from build123d import *

# Parameters (mm, degrees)
SKETCH1_W                = 135
SKETCH1_H                = 20
BOSS_EXTRUDE1_DEPTH      = 3
BOSS_EXTRUDE2_START      = -20
BOSS_EXTRUDE2_DEPTH      = 20
SKETCH5_R                = 1.6
CUT_EXTRUDE1_DEPTH       = 5
BOSS_EXTRUDE3_DEPTH      = 2.7
SKETCH7_W                = 5
SKETCH7_H                = 2.576431393
BOSS_EXTRUDE4_DEPTH      = 20
SKETCH9_W                = 5
SKETCH9_H                = 2.400677448
SKETCH9_H_2              = 2.137863312
BOSS_EXTRUDE5_DEPTH      = 18
SKETCH10_R               = 1.51
CUT_EXTRUDE2_DEPTH       = 46
SKETCH11_W               = 87
SKETCH11_H               = 20
CUT_EXTRUDE3_DEPTH       = 7
BOSS_EXTRUDE7_DEPTH      = 26.162
BOSS_EXTRUDE7_DEPTH_BACK = 3
SKETCH12_W               = 9.518804698
SKETCH12_H               = 20
SKETCH13_R               = 1.6
CUT_EXTRUDE4_DEPTH       = 36.162
BOSS_EXTRUDE8_DEPTH      = 4
FILLET1_R                = 10
SKETCH18_R               = 1.6
CUT_EXTRUDE6_DEPTH       = 4


# Read off the part's stored shape, not the designer's step: Boss-Extrude2
with BuildPart() as part:
    # Sketch1 → Boss-Extrude1 (new body)
    with BuildSketch(Plane(origin=(0, 0, 0), x_dir=(1, 0, 0), z_dir=(0, 1, 0))):
        with Locations((67.5, 10)):
            Rectangle(SKETCH1_W, SKETCH1_H)
    extrude(amount=BOSS_EXTRUDE1_DEPTH)


with BuildPart() as body_2:
    # Boss-Extrude2 outline → Boss-Extrude2 (new body)
    with BuildSketch(Plane(origin=(0, 0, -20), x_dir=(-1, 0, 0), z_dir=(0, 0, -1)).offset(BOSS_EXTRUDE2_START)):
        Polygon((-135, 0), (0, 0), (0, -26.161397266), (8, -26.161397266), (8, -23.458863774), (2.440744198, -23.458863774), (2.440744198, 3), (-135, 3), align=None)
    extrude(amount=BOSS_EXTRUDE2_DEPTH)

    # Sketch5 → Cut-Extrude1 (cut)
    with BuildSketch(Plane(origin=(0, -26.161397266, 0), x_dir=(-1, 0, 0), z_dir=(0, -1, 0))):
        with Locations(Location((4.475005096, 14.904630263, 0), (0, 0, 90))):
            Circle(SKETCH5_R)
        with Locations(Location((4.475005096, 4.904630263, 0), (0, 0, 90))):
            Circle(SKETCH5_R)
    extrude(amount=-CUT_EXTRUDE1_DEPTH, mode=Mode.SUBTRACT)

    # Sketch6 → Boss-Extrude3 (add)
    with BuildSketch(Plane(origin=(0, -26.161397266, 0), x_dir=(-1, 0, 0), z_dir=(0, -1, 0))):
        Polygon((0, 26.189005721), (0, 20), (8, 20), (8, 23.612574328), (17, 23.612574328), (17, 26.189005721), align=None)
    extrude(amount=-BOSS_EXTRUDE3_DEPTH)

    # Sketch7 → Boss-Extrude4 (add)
    with BuildSketch(Plane.XZ.offset(26.161397266)):
        with Locations((-14.5, -24.900790025)):
            Rectangle(SKETCH7_W, SKETCH7_H)
    extrude(amount=BOSS_EXTRUDE4_DEPTH)

    # Sketch9 → Boss-Extrude5 (add)
    with BuildSketch(Plane.XY.offset(-23.612574328)):
        with Locations((-14.5, -44.961058542)):
            Rectangle(SKETCH9_W, SKETCH9_H)
        with Locations((-14.5, -37.813107102)):
            Rectangle(SKETCH9_W, SKETCH9_H_2)
    extrude(amount=BOSS_EXTRUDE5_DEPTH)

    # Sketch10 → Cut-Extrude2 (cut)
    with BuildSketch(Plane(origin=(0, -46.161397266, 0), x_dir=(-1, 0, 0), z_dir=(0, -1, 0))):
        with Locations(Location((14.400768804, 9.736347936, 0), (0, 0, 90))):
            Circle(SKETCH10_R)
    extrude(amount=-CUT_EXTRUDE2_DEPTH, mode=Mode.SUBTRACT)


with BuildPart() as cut_extrude3_tool:
    # Sketch11 → Cut-Extrude3 (new body)
    with BuildSketch(Plane.XZ):
        with Locations((91.5, -10)):
            Rectangle(SKETCH11_W, SKETCH11_H)
    extrude(amount=-CUT_EXTRUDE3_DEPTH)


with BuildPart() as part_1:
    add(part.part)

    # Cut-Extrude3: cut by cut_extrude3_tool
    add(cut_extrude3_tool.part, mode=Mode.SUBTRACT)



with BuildPart() as body_2_1:
    add(body_2.part)

    # Cut-Extrude3: cut by cut_extrude3_tool
    add(cut_extrude3_tool.part, mode=Mode.SUBTRACT)


with BuildPart() as part_2:
    add(part_1.part)

    add(body_2_1.part)  # Boss-Extrude7 merges body 2
    # Sketch12 → Boss-Extrude7 (add, two sides: drawn at the far end of the back side and taken through both)
    with BuildSketch(Plane(origin=(0, 0, 0), x_dir=(-1, 0, 0), z_dir=(0, -1, 0)).offset(-BOSS_EXTRUDE7_DEPTH_BACK)):
        with Locations((-45.240597651, 10)):
            Rectangle(SKETCH12_W, SKETCH12_H)
    extrude(amount=BOSS_EXTRUDE7_DEPTH + BOSS_EXTRUDE7_DEPTH_BACK)

    # Sketch13 → Cut-Extrude4 (cut)
    with BuildSketch(Plane(origin=(0, -26.162, 0), x_dir=(-1, 0, 0), z_dir=(0, -1, 0))):
        with Locations(Location((-45.024994904, 4.904630263, 0), (0, 0, 90))):
            Circle(SKETCH13_R)
        with Locations(Location((-45.024994904, 14.904630263, 0), (0, 0, 90))):
            Circle(SKETCH13_R)
    extrude(amount=-CUT_EXTRUDE4_DEPTH, mode=Mode.SUBTRACT)

    # Sketch14 → Boss-Extrude8 (add)
    with BuildSketch(Plane(origin=(0, 3, 0), x_dir=(1, 0, 0), z_dir=(0, 1, 0))):
        Polygon((50, 20), (50, 0), (148.480775301, 17.298817767), (148.480775301, 37.364817767), align=None)
    extrude(amount=-BOSS_EXTRUDE8_DEPTH)

    # Fillet1
    # the kernel refuses this fillet: 10 mm, written as the material it takes off along each edge
    with BuildSketch(Plane(origin=(148.480775301, 23.991341286, -17.298817767), x_dir=(-0.9849204245014849, 0, 0.1730079691800782), z_dir=(0, -1, 0))) as fillet1_piece_1:
        with BuildLine():
            CenterArc((FILLET1_R * 0.83965365145, FILLET1_R), FILLET1_R, 189.96275502, 80.03724498)
            Line((-FILLET1_R * 0.145266773052, FILLET1_R * 0.82699203082), (0, 0))
            Line((0, 0), (FILLET1_R * 0.83965365145, 0))
        make_face()
    extrude(amount=45.982682572, mode=Mode.SUBTRACT)
    with BuildSketch(Plane(origin=(148.480775301, 32.793839815, -37.364817767), x_dir=(0, 0, 1), z_dir=(0, -1, 0))) as fillet1_piece_2:
        with BuildLine():
            CenterArc((FILLET1_R * 1.19175359259, FILLET1_R), FILLET1_R, 170, 100)
            Line((FILLET1_R * 0.206945839582, FILLET1_R * 1.17364817767), (0, 0))
            Line((0, 0), (FILLET1_R * 1.19175359259, 0))
        make_face()
    extrude(amount=63.58767963, mode=Mode.SUBTRACT)

    # Sketch18 → Cut-Extrude6 (cut)
    with BuildSketch(Plane(origin=(0, 3, 0), x_dir=(1, 0, 0), z_dir=(0, 1, 0))):
        with Locations(Location((138.480775301, 25.447281841, 0), (0, 0, 270))):
            Circle(SKETCH18_R)
        with Locations(Location((119.473985668, 22.095872012, 0), (0, 0, 270))):
            Circle(SKETCH18_R)
        with Locations(Location((110.610715891, 20.533038413, 0), (0, 0, 270))):
            Circle(SKETCH18_R)
        with Locations(Location((129.617505524, 23.884448242, 0), (0, 0, 270))):
            Circle(SKETCH18_R)
    extrude(amount=-CUT_EXTRUDE6_DEPTH, mode=Mode.SUBTRACT)


solid = part_2.part
Could you check a few things on this model? Use its own coordinates, in mm. A direction names the side the tool comes from. Give positions to 0.01 mm unless a question says otherwise; leave off trailing zeros. Write each loop counter-clockwise with the first axis right and the second up, starting at its lowest first coordinate (ties: lowest second). Pieces come first, ordered by that corner, then holes. Notation, with made-up numbers: (86, 64.5) -> (112, 64.5) arc R11 cw to (112, 78.5) -> close; hole circle Ø5 at (53, 5). An arc over 180 degrees is marked (long way). Answer as a JSON object with one key per item and string values.
Q1. We'd pull the mould along Z, two halves only. Please class faces 4 (the cylindrical face through (144.8, 1, -33.2)), 5 (the flat face through (-14, -29, -23.613)), 6 (the cylindrical face through (130.1, 1.03, -22.36)): released by +Z, released by -Z, zero draft, split by the parting line, or undercut.
Taken from the geometry:
{"face 4": "released by -Z", "face 5": "released by +Z", "face 6": "undercut"}
Q2. Which directions (+Z, -Z, +X, -X, +Y, -Y) give clear straight access to the entire face, cutting with the end or side of a thin tool? Please do faces 1 (the flat face through (-5, -23.459, -10)), 2 (the flat face through (-6, -23.461, -24)), 3 (the flat face through (-12, -38, -18)).
Taken from the geometry:
{"face 1": "+Z, -Z, -X, +Y", "face 2": "-Z, +X, -X, +Y", "face 3": "+Z, -Z, +X, -Y"}
Q3. Suppose I cut it at B-B on x = 11.5. Write out the boundary of the cut face in (y, z), then the cut area to 3 significant figures.
Taken from the geometry:
{"outline": "(0, -20) -> (3, -20) -> (3, 0) -> (0, 0) -> close", "area": "60.0 mm²"}
Q4. Suppose I cut it at A-A on y = -21. Write out the boundary of the cut face in (x, z) (3 decimals), then the cut area to 3 significant figures.
Taken from the geometry:
{"outline": "(-2.441, -20) -> (0, -20) -> (0, 0) -> (-2.441, 0) -> close; (40.481, -20) -> (50, -20) -> (50, 0) -> (40.481, 0) -> close; hole circle Ø3.2 at (45.025, -14.905); hole circle Ø3.2 at (45.025, -4.905)", "area": "223 mm²"}
Q5. Will these pins go through, and if not, where does the flat tip stop? pin 1 Ø2 at (y, z) = (-39.5, -18.5) entering from +X; pin 2 Ø1.9 at (x, z) = (119.47, -22.1) entering from +Y; pin 3 Ø21 at (y, z) = (-7.5, -13.5) entering from +X; pin 4 Ø4 at (x, z) = (-13.5, -11.5) entering from +Y.
Taken from the geometry:
{"pin 1": "stops at x = -12", "pin 2": "passes through", "pin 3": "stops at x = 147.67", "pin 4": "stops at y = -36.74"}
Q6. Please list where these lines run through material, in increasing order: L1, parallel to X at y = -18, z = -1.5; L2, parallel to Y at x = -5.5, z = -10; L3, parallel to Y at x = 14.5, z = -5.
Taken from the geometry:
{"L1": "x = -2.44 to 0, 40.48 to 50", "L2": "y = -26.16 to -23.46", "L3": "y = 0 to 3"}
Q7. Suppose I cut it at C-C on z = -28.5. Write out the boundary of the cut face in (x, y), then the cut area to 3 significant figures.
Taken from the geometry:
{"outline": "(98.21, -1) -> (148, -1) -> (148, 3) -> (98.21, 3) -> close", "area": "199 mm²"}
